Answer from the drawing. Dimensions are ordinates in mm from the lowest x, y and z of the part. A direction names the side the tool comes from. Coordinates: 2 decimals unless noted, no trailing zeros. Loops run counter-clockwise (first coordinate to the right, second up) from the corner with the lowest first, then second, coordinate; pieces in that order, holes last. Notation, with made-up numbers: M -12,-21.75 L 21,-21.75 A14 ccw 21,-17.75 Z; hole C -8,7.5 d6. An arc over 180 degrees is marked long. One line per item, written item: value. Start each with the question number.
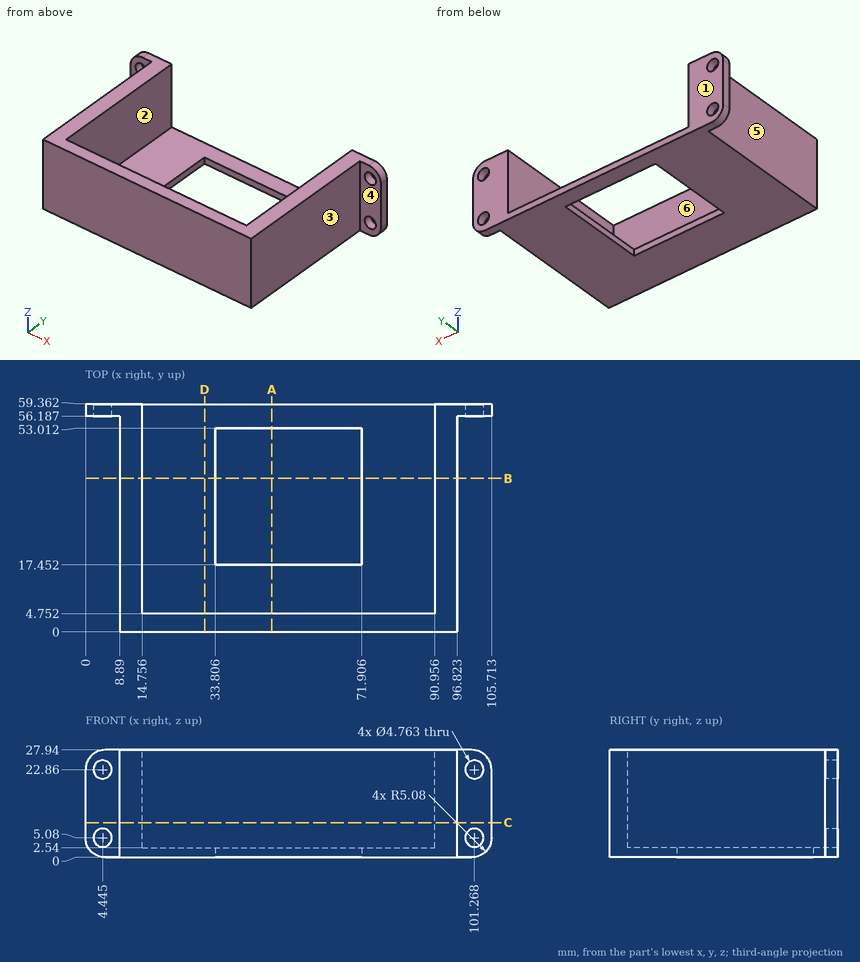
1) For a pull along X with two mould halves and no side action, classify the marked faces 1, 2 and 3 as released by +X, released by -X, zero draft, split by the parting line, or undercut.
2) Section B-B (y = 40) is taken. Determine the outline of the cut face in (x, z).
3) Section D-D (x = 31) is taken. Determine the outline of the cut face in (y, z).
4) Section C-C (z = 9) is taken. Determine the outline of the cut face in (x, y).
5) Consider line 1 along X through (y, z) = (52.5, 4); line 2 along X through (y, z) = (42, 1.5); line 3 along Y through (x, z) = (42, 2). Determine where each line is inside the solid, lowest interval first.
6) A tool of negligible diameter and unlimited length cuts with its end or side. For the marked faces 4, 5 and 6, from which of +Z, -Z, +X, -X, +Y, -Y can it reach the whole face along a straight path? Write none if from no direction.
7) Flat-ended cylindrical pins translate along their axes: pin 1 (2.5 mm diameter, centred on x = 6, z = 16.5, fed in from -Y); pin 2 (4 mm diameter, centred on x = 35, z = 14.5, fed in from +Y); pin 3 (2 mm diameter, centred on y = 40, z = 1, fed in from -X). Find the tip coordinate at first contact, or state that the pin passes through.
8) Section A-A (x = 48.5) is taken. Determine the outline of the cut face in (y, z).
Results found:
1. face 1: zero draft
1. face 2: undercut
1. face 3: released by +X
2. outline: M 8.89,0 L 33.81,0 L 33.81,2.54 L 14.76,2.54 L 14.76,27.94 L 8.89,27.94 Z; M 71.91,0 L 96.82,0 L 96.82,27.94 L 90.96,27.94 L 90.96,2.54 L 71.91,2.54 Z
3. outline: M 0,0 L 59.36,0 L 59.36,2.54 L 4.75,2.54 L 4.75,27.94 L 0,27.94 Z
4. outline: M 0,56.19 L 8.89,56.19 L 8.89,0 L 96.82,0 L 96.82,56.19 L 105.71,56.19 L 105.71,59.36 L 90.96,59.36 L 90.96,4.75 L 14.76,4.75 L 14.76,59.36 L 0,59.36 Z
5. line 1: x = 8.89 to 14.76, 90.96 to 96.82
5. line 2: x = 8.89 to 33.81, 71.91 to 96.82
5. line 3: y = 0 to 17.45, 53.01 to 59.36
6. face 4: +Z, -Z, +X, -Y
6. face 5: +Z, -Z, -X, -Y
6. face 6: +Z, +Y
7. pin 1: stops at y = 56.19
7. pin 2: stops at y = 4.75
7. pin 3: stops at x = 8.89
8. outline: M 0,0 L 17.45,0 L 17.45,2.54 L 4.75,2.54 L 4.75,27.94 L 0,27.94 Z; M 53.01,0 L 59.36,0 L 59.36,2.54 L 53.01,2.54 Z
